from build123d import *

# Parameters (mm, degrees)
SKETCH1_R           = 14.2875
SKETCH1_R_2         = 2.54
BOSS_EXTRUDE1_DEPTH = 3.175
FILLET1_R           = 3.175


with BuildPart() as part:
    # Sketch1 → Boss-Extrude1 (new body)
    with BuildSketch(Plane.XY):
        with BuildLine():
            Line((0, 0), (152.4, 0))
            Line((152.4, 0), (152.4, 25.4))
            Line((152.4, 25.4), (123.236852256, 52.859492597))
            ThreePointArc((123.236852256, 52.859492597), (116.759751152, 56.979103271), (109.22, 58.42))
            Line((109.22, 58.42), (43.18, 58.42))
            ThreePointArc((43.18, 58.42), (35.640248848, 56.979103271), (29.163147744, 52.859492597))
            Line((29.163147744, 52.859492597), (0, 25.4))
            Line((0, 25.4), (0, 0))
        make_face()
        with Locations((43.18, 37.973)):
            Circle(SKETCH1_R, mode=Mode.SUBTRACT)
        with Locations((109.22, 37.973)):
            Circle(SKETCH1_R, mode=Mode.SUBTRACT)
        with Locations((12.7, 12.7)):
            Circle(SKETCH1_R_2, mode=Mode.SUBTRACT)
        with Locations((139.7, 12.7)):
            Circle(SKETCH1_R_2, mode=Mode.SUBTRACT)
    extrude(amount=BOSS_EXTRUDE1_DEPTH)

    # Fillet1
    fillet1_edges = [part.edges().sort_by_distance(p)[0] for p in [
        (0, 25.4, 1.5875),
        (152.4, 25.4, 1.5875),
        (152.4, 0, 1.5875),
        (0, 0, 1.5875),
    ]]
    fillet(fillet1_edges, radius=FILLET1_R)


solid = part.part
Check sheet for the modelled part. Datum: model origin and axes. Units: mm. Round coordinates to 2 decimals unless told otherwise and drop trailing zeros. Loops run counter-clockwise (first coordinate to the right, second up) from the corner with the lowest first, then second, coordinate; pieces in that order, holes last. Notation, with made-up numbers: (-0.75, -7.5) -> (8.25, -7.5) arc R26 ccw to (8.25, 11.5) -> close; hole circle Ø1 at (-37, 72.25). An arc over 180 degrees is marked (long way). Put each result on its own line as item: value. Start each with the question number.
1. Scan lines: probe 1 along X at (y, z) = (14, 2.6); probe 2 along Y at (x, z) = (43.18, 1.6); probe 3 along X at (y, z) = (12, 0.6). Record each from-to range of solid material in increasing order.
2. Section check C-C (z = 2.6). Give the number of separate pieces and of enclosed holes in the cut face, plus the area to 3 significant figures.
3. Gauge pin test, flat ends, axial feed: pin 1 (1 mm diameter, centred on y = 49.5, z = 2, fed in from -X); pin 2 (1 mm diameter, centred on y = 43.5, z = 1, fed in from +X). Record the tip position at first contact, or that the pin passes through.
4. Section check A-A (x = 115). Enter the section's corners in (y, z) (3 decimals).
5. Section check D-D (y = 47). Enter the section's corners in (x, z) (3 decimals).
6. Section check B-B (y = 12.7). Enter the section's corners in (x, z) (3 decimals).
7. Draft check along X on faces 1 (the face through (116.86, 56.94, 1.57)), 2 (the face through (122.85, 42.26, 1.57)), 3 (the face through (75, 0, 2)). Enter one of: +X half, -X half, draft (parallel to the pull), parting line (faces both ways), or undercut.
Findings:
1. probe 1: x = 0 to 10.52, 14.88 to 137.52, 141.88 to 152.4
1. probe 2: y = 0 to 23.69, 52.26 to 58.42
1. probe 3: x = 0 to 10.26, 15.14 to 137.26, 142.14 to 152.4
2. separate pieces: 1
2. enclosed holes: 4
2. area: 6,400 mm^2
3. pin 1: stops at x = 25.06
3. pin 2: stops at x = 133.71
4. outline: (0, 0) -> (24.907, 0) -> (24.907, 3.175) -> (0, 3.175) -> close; (51.039, 0) -> (57.586, 0) -> (57.586, 3.175) -> (51.039, 3.175) -> close
5. outline: (22.94, 0) -> (32.105, 0) -> (32.105, 3.175) -> (22.94, 3.175) -> close; (54.255, 0) -> (98.145, 0) -> (98.145, 3.175) -> (54.255, 3.175) -> close; (120.295, 0) -> (129.46, 0) -> (129.46, 3.175) -> (120.295, 3.175) -> close
6. outline: (0, 0) -> (10.16, 0) -> (10.16, 3.175) -> (0, 3.175) -> close; (15.24, 0) -> (137.16, 0) -> (137.16, 3.175) -> (15.24, 3.175) -> close; (142.24, 0) -> (152.4, 0) -> (152.4, 3.175) -> (142.24, 3.175) -> close
7. face 1: +X half
7. face 2: undercut
7. face 3: draft
